```python
from build123d import *

# Parameters (mm, degrees)
F1_DEPTH = 20
F2_ANGLE = -90


with BuildPart() as f1:
    # F0 (on Front) → F1 (new body)
    with BuildSketch(Plane.XZ):
        Polygon((-10.0444195345, 6.7202923819), (-7.0444195345, 6.7202923819), (-7.0444195345, -22.0063235611), (0, -22.0063235611), (2.1582664922, -22.0060478896), (2, -15.5988996848), (0, -15.5988996848), (0, -20.1908871531), (-4, -20.1908871531), (-4, 9.0697817504), (-12.0444195345, 9.0697817504), (-12.0444195345, 0), (-10.0444195345, 0), align=None)
    extrude(amount=F1_DEPTH)


with BuildPart() as f1_1:
    # F2: moved
    add(f1.part.rotate(Axis((-2, -20, -20.1908871531), (1, 0, 0)), F2_ANGLE))


solid = f1_1.part
```
Design review of the part built by this model. Coordinates are the model's own, in mm. A direction names the side the tool comes from. Coordinates: 2 decimals unless noted, no trailing zeros. Order: outer loops, then holes, each group sorted by start corner. A loop starts at its lowest first (then second) coordinate and runs counter-clockwise, first axis right, second up.
1) For faces 1 (the flat face through (0, -18, -30)), 2 (the flat face through (-6, -5, -20.191)), 3 (the flat face through (-11, 0.191, -30)), 4 (the flat face through (-7.044, -7, -30)), 5 (the flat face through (1, -15.408, -30)), list the 3-axis set-ups (+Z, -Z, +X, -X, +Y, -Y) from which the entire face can be reached by the end or side of a thin tool; tool diameter is ignored.
2) Take a section at D-D, the plane x = -8. Give the boundary of the cut face in (y, z), and give its area (3 significant figures).
3) Take a section at C-C, the plane y = -17.5. Give the boundary of the cut face in (x, z), and give its area (3 significant figures).
4) Wall thickness on line 1 along X through (y, z) = (5, -31.5); line 2 along X through (y, z) = (7, -21); line 3 along X through (y, z) = (-14.5, -22.5): over which ranges is each line inside the solid? List them lowest first.
5) Mouldability with a two-part tool opening along X and no side actions: class faces 6 (the flat face through (-12.044, 5, -30)), 7 (the flat face through (-8, 9.261, -30)), 8 (the flat face through (-2, -20, -30)) as +X half, -X half, draft (parallel to the pull), parting line (faces both ways), or undercut.
6) Clearance check with flat-ended pins moving along their axes: pin 1 (3 mm diameter, centred on y = 3, z = -25, fed in from +X); pin 2 (1.2 mm diameter, centred on x = -2, z = -30, fed in from +Y); pin 3 (6 mm diameter, centred on y = -4, z = -27.5, fed in from -X). State where each tip first meets the part, or that it passes through.
7) Take a section at A-A, the plane y = 6.5. Give the boundary of the cut face in (x, z).
8) Take a section at B-B, the plane z = -37.75. Give the boundary of the cut face in (x, y), and give its area (3 significant figures).
Returned:
1. face 1: +Z, -Z, +Y
1. face 2: +Z, +X, -X, +Y, -Y
1. face 3: +Z, -Z, -X, -Y
1. face 4: +Z, -Z, -Y
1. face 5: +Z, -Z, +X, +Y
2. outline: (6.91, -40.19) - (9.26, -40.19) - (9.26, -20.19) - (6.91, -20.19) - close
2. area: 47.0 mm2
3. outline: (-7.04, -40.19) - (-4, -40.19) - (-4, -20.19) - (-7.04, -20.19) - close; (0, -40.19) - (2.05, -40.19) - (2.05, -20.19) - (0, -20.19) - close
3. area: 102 mm2
4. line 1: x = -12.04 to -10.04, -7.04 to -4
4. line 2: x = -12.04 to -4
4. line 3: x = -7.04 to -4
5. face 6: -X half
5. face 7: draft
5. face 8: undercut
6. pin 1: stops at x = -4
6. pin 2: stops at y = -20
6. pin 3: stops at x = -7.04
7. outline: (-12.04, -40.19) - (-10.04, -40.19) - (-10.04, -20.19) - (-12.04, -20.19) - close; (-7.04, -40.19) - (-4, -40.19) - (-4, -20.19) - (-7.04, -20.19) - close
8. outline: (-12.04, 0.19) - (-10.04, 0.19) - (-10.04, 6.91) - (-7.04, 6.91) - (-7.04, -21.82) - (0, -21.82) - (2.16, -21.82) - (2, -15.41) - (0, -15.41) - (0, -20) - (-4, -20) - (-4, 9.26) - (-12.04, 9.26) - close
8. area: 140 mm2
